```python
from build123d import *

# Parameters (mm, degrees)
BOSS_EXTRUDE1_DEPTH             = 207
SKETCH9_R                       = 2.5
BOSS_EXTRUDE2_DEPTH             = 3
BOSS_EXTRUDE3_DEPTH             = 9
BOSS_EXTRUDE3_DEPTH_BACK        = 9
SKETCH10_R                      = 21
SKETCH10_R_2                    = 18.5
CUT_EXTRUDE1_DEPTH              = 19
CUT_EXTRUDE1_DEPTH_BACK         = 19
F_3_0MM_DOWEL_HOLE1_D           = 3
F_3_0MM_DOWEL_HOLE1_DEPTH       = 7.5
F_3_0MM_DOWEL_HOLE1_CSINK_D     = 3.05
F_3_0MM_DOWEL_HOLE1_CSINK_ANGLE = 90
F_3_0MM_DOWEL_HOLE1_TIP         = 0.901290929
FILLET1_R                       = 5
SKETCH13_W                      = 19.825171118
SKETCH13_H                      = 19.672097988
CUT_EXTRUDE2_DEPTH              = 10
F_2_5MM_DOWEL_HOLE1_D           = 2.5
F_2_5MM_DOWEL_HOLE1_CSINK_D     = 2.55
F_2_5MM_DOWEL_HOLE1_CSINK_ANGLE = 90


with BuildPart() as part:
    # Sketch2 → Boss-Extrude1 (new body)
    with BuildSketch(Plane(origin=(0, 0, 0), x_dir=(0, 0, -1), z_dir=(1, 0, 0))):
        with BuildLine():
            Line((-8, 15), (8, 15))
            ThreePointArc((8, 15), (9.414213562, 14.414213562), (10, 13))
            Line((10, 13), (10, -13))
            ThreePointArc((10, -13), (9.414213562, -14.414213562), (8, -15))
            Line((8, -15), (-8, -15))
            ThreePointArc((-8, -15), (-9.414213562, -14.414213562), (-10, -13))
            Line((-10, -13), (-10, 13))
            ThreePointArc((-10, 13), (-9.414213562, 14.414213562), (-8, 15))
        make_face()
        with BuildLine():
            Line((-7, 14), (7, 14))
            ThreePointArc((7, 14), (8.414213562, 13.414213562), (9, 12))
            Line((9, 12), (9, -12))
            ThreePointArc((9, -12), (8.414213562, -13.414213562), (7, -14))
            Line((7, -14), (-7, -14))
            ThreePointArc((-7, -14), (-8.414213562, -13.414213562), (-9, -12))
            Line((-9, -12), (-9, 12))
            ThreePointArc((-9, 12), (-8.414213562, 13.414213562), (-7, 14))
        make_face(mode=Mode.SUBTRACT)
    extrude(amount=BOSS_EXTRUDE1_DEPTH)

    # Sketch9 → Boss-Extrude2 (add)
    # profile 1 of 2: a face of its own
    with BuildSketch(Plane(origin=(207, 0, 0), x_dir=(0, 0, -1), z_dir=(1, 0, 0))):
        with BuildLine():
            Line((0, -5), (0, -20))
            Line((0, -20), (30, -20))
            Line((30, -20), (30, 20))
            Line((30, 20), (0, 20))
            Line((0, 20), (0, 5))
            ThreePointArc((0, 5), (3.535533906, 3.535533906), (5, 0))
            ThreePointArc((5, 0), (3.535533906, -3.535533906), (0, -5))
        make_face()
        with Locations((23, -13)):
            Circle(SKETCH9_R, mode=Mode.SUBTRACT)
        with Locations((23, 13)):
            Circle(SKETCH9_R, mode=Mode.SUBTRACT)
    # profile 2 of 2: a face of its own
    with BuildSketch(Plane(origin=(207, 0, 0), x_dir=(0, 0, -1), z_dir=(1, 0, 0))):
        with BuildLine():
            Line((-30, 20), (-30, -20))
            Line((-30, -20), (0, -20))
            Line((0, -20), (0, -5))
            ThreePointArc((0, -5), (-5, 0), (0, 5))
            Line((0, 5), (0, 20))
            Line((0, 20), (-30, 20))
        make_face()
        with Locations((-23, -13)):
            Circle(SKETCH9_R, mode=Mode.SUBTRACT)
        with Locations((-23, 13)):
            Circle(SKETCH9_R, mode=Mode.SUBTRACT)
    extrude(amount=-BOSS_EXTRUDE2_DEPTH)

    # Sketch10 → Boss-Extrude3 (add, two sides: drawn at the far end of the back side and taken through both)
    # profile 1 of 3: a face of its own
    with BuildSketch(Plane.XY.offset(-BOSS_EXTRUDE3_DEPTH_BACK)):
        Circle(SKETCH10_R)
        Circle(SKETCH10_R_2, mode=Mode.SUBTRACT)
    # profile 2 of 3: a face of its own
    with BuildSketch(Plane.XY.offset(-BOSS_EXTRUDE3_DEPTH_BACK)):
        with BuildLine():
            ThreePointArc((10.828203914, 15), (0, 18.5), (-10.828203914, 15))
            Line((-10.828203914, 15), (10.828203914, 15))
        make_face()
    # profile 3 of 3: a face of its own
    with BuildSketch(Plane.XY.offset(-BOSS_EXTRUDE3_DEPTH_BACK)):
        with BuildLine():
            ThreePointArc((-10.828203914, -15), (0, -18.5), (10.828203914, -15))
            Line((10.828203914, -15), (-10.828203914, -15))
        make_face()
    extrude(amount=BOSS_EXTRUDE3_DEPTH + BOSS_EXTRUDE3_DEPTH_BACK)

    # Sketch10_3 → Cut-Extrude1 (cut, two sides: drawn at the far end of the back side and taken through both)
    with BuildSketch(Plane.XY.offset(-CUT_EXTRUDE1_DEPTH_BACK)):
        with BuildLine():
            Line((-10.828203914, -15), (10.828203914, -15))
            ThreePointArc((10.828203914, -15), (16.470758519, -8.42402005), (18.5, 0))
            ThreePointArc((18.5, 0), (16.470758519, 8.42402005), (10.828203914, 15))
            Line((10.828203914, 15), (-10.828203914, 15))
            ThreePointArc((-10.828203914, 15), (-18.5, 0), (-10.828203914, -15))
        make_face()
    extrude(amount=CUT_EXTRUDE1_DEPTH + CUT_EXTRUDE1_DEPTH_BACK, mode=Mode.SUBTRACT)

    # 3.0mm Dowel Hole1
    with Locations(Plane(origin=(0, -15, 0), x_dir=(1, 0, 0), z_dir=(0, 1, 0))):
        with Locations((0, 0)):
            CounterSinkHole(F_3_0MM_DOWEL_HOLE1_D / 2, F_3_0MM_DOWEL_HOLE1_CSINK_D / 2, depth=F_3_0MM_DOWEL_HOLE1_DEPTH, counter_sink_angle=F_3_0MM_DOWEL_HOLE1_CSINK_ANGLE)
            with Locations((0, 0, -(F_3_0MM_DOWEL_HOLE1_DEPTH + F_3_0MM_DOWEL_HOLE1_TIP / 2))):  # 118° drill point
                Cone(0, F_3_0MM_DOWEL_HOLE1_D / 2, F_3_0MM_DOWEL_HOLE1_TIP, mode=Mode.SUBTRACT)

    # Fillet1
    fillet1_edges = [part.edges().sort_by_distance(p)[0] for p in [
        (205.5, -20, 30),
        (205.5, 20, 30),
        (205.5, 20, -30),
        (205.5, -20, -30),
    ]]
    fillet(fillet1_edges, radius=FILLET1_R)

    # Sketch13 → Cut-Extrude2 (cut)
    with BuildSketch(Plane(origin=(0, -20, 0), x_dir=(1, 0, 0), z_dir=(0, 1, 0))):
        Rectangle(SKETCH13_W, SKETCH13_H)
    extrude(amount=-CUT_EXTRUDE2_DEPTH, mode=Mode.SUBTRACT)

    # 2.5mm Dowel Hole1 (through all)
    with Locations(Plane.XY.offset(10)):
        with Locations((65, 0), (175, 0)):
            CounterSinkHole(F_2_5MM_DOWEL_HOLE1_D / 2, F_2_5MM_DOWEL_HOLE1_CSINK_D / 2, counter_sink_angle=F_2_5MM_DOWEL_HOLE1_CSINK_ANGLE)


solid = part.part
```
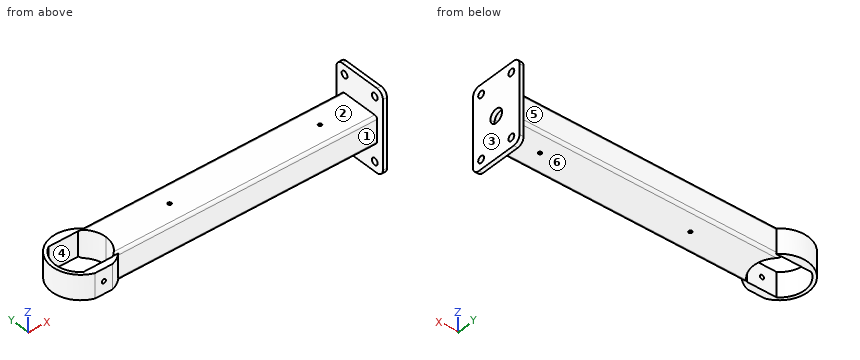
Model file for the job. Use its own axes, mm. Face numbers are marked on the shaded views. A direction names the side the tool comes from. Round coordinates to 2 decimals unless told otherwise and drop trailing zeros. Write each loop counter-clockwise with the first axis right and the second up, starting at its lowest first coordinate (ties: lowest second). Pieces come first, ordered by that corner, then holes. Notation, with made-up numbers: (51, 80) - (60, 80) arc R28 cw to (60, 112) - close; hole circle Ø10 at (13.25, 42.25). An arc over 180 degrees is marked (long way). One line per item, written item: value.
(1) 3-axis set-ups, long thin cutter, end or side, ignore diameter. For the marked faces 4, 5 and 6: which of +Z, -Z, +X, -X, +Y, -Y reach the whole face in a straight line?
Values follow:
face 4: +Z, -Z
face 5: +Z, -Z, +Y
face 6: -Z, -X, +Y, -Y
(2) Two-plate mould, pull along X, no slides. Class the marked faces 1, 2 and 3: pulls with the +X half, pulls with the -X half, needs draft (parallel to the pull), parting line crosses it, or undercut.
Values follow:
face 1: undercut
face 2: needs draft
face 3: pulls with the +X half
(3) Cut at D-D, the plane y = 8. Give the cut face in (x, z).
Values follow:
outline: (-19.42, -9) - (-16.68, -9) - (-16.68, 9) - (-19.42, 9) - close; (16.68, -10) - (204, -10) - (204, -30) - (207, -30) - (207, 30) - (204, 30) - (204, 10) - (16.68, 10) - close; hole (19.42, -9) - (204, -9) - (204, 9) - (19.42, 9) - close
(4) Cut at A-A, the plane x = 107.5. Give the cut face in (y, z).
Values follow:
outline: (-15, -8) arc R2 ccw to (-13, -10) - (13, -10) arc R2 ccw to (15, -8) - (15, 8) arc R2 ccw to (13, 10) - (-13, 10) arc R2 ccw to (-15, 8) - close; hole (-14, -7) arc R2 ccw to (-12, -9) - (12, -9) arc R2 ccw to (14, -7) - (14, 7) arc R2 ccw to (12, 9) - (-12, 9) arc R2 ccw to (-14, 7) - close
(5) Cut at C-C, the plane y = 18. Give the cut face in (x, z).
Values follow:
outline: (-10.82, -9) - (10.82, -9) - (10.82, 9) - (-10.82, 9) - close; (204, -29) - (207, -29) - (207, 29) - (204, 29) - close
(6) Cut at B-B, the plane z = -23. Give the cut face in (x, y), plus the area to 3 significant figures.
Values follow:
outline: (204, -20) - (207, -20) - (207, -15.5) - (204, -15.5) - close; (204, -10.5) - (207, -10.5) - (207, 10.5) - (204, 10.5) - close; (204, 15.5) - (207, 15.5) - (207, 20) - (204, 20) - close
area: 90.0 mm²
(7) Drop flat-ended pins along their axis: P1, Ø19, axis at x = 114.5, y = -3.5, coming from the +Z side; P2, Ø1.8, axis at x = 0, z = 0, coming from the -Y side; P3, Ø5, axis at x = 95, z = -2, coming from the -Y side; P4, Ø12, axis at y = -1, z = 12.5, coming from the -X side. Give the stop position or say it passes through.
Values follow:
P1: stops at z = 10
P2: stops at y = 15
P3: stops at y = -15
P4: stops at x = -21
(8) Wall check: probe 1 along Y at (x, z) = (205.3, -23); probe 2 along Z at (x, y) = (136, -4); probe 3 along X at (y, z) = (18, -3). Give the ranges that are in metal, low to high.
Values follow:
probe 1: y = -20 to -15.5, -10.5 to 10.5, 15.5 to 20
probe 2: z = -10 to -9, 9 to 10
probe 3: x = -10.82 to 10.82, 204 to 207
